The model under review builds one solid part; all positions refer to its coordinate system, in mm. Face numbers are marked on the shaded views. A direction names the side the tool comes from. Coordinates: 2 decimals unless noted, no trailing zeros. Order: outer loops, then holes, each group sorted by start corner. A loop starts at its lowest first (then second) coordinate and runs counter-clockwise, first axis right, second up. Notation, with made-up numbers: M -19.75,40.5 L 15.25,40.5 A31 cw 15.25,65.5 Z; hole C 47.25,45.5 d7. An arc over 180 degrees is marked long. One line per item, written item: value.
```python
from build123d import *

# Parameters (mm, degrees)
SKETCH_1_R          = 1.5
EXTRUDE_1_DEPTH     = 6
SKETCH_2_R          = 3.5
EXTRUDE_2_DEPTH     = 1.8
CUT_EXTRUDE_1_DEPTH = 1
FILLET_1_R          = 1


with BuildPart() as part:
    # 草图1 → 凸台-拉伸1 (new body)
    with BuildSketch(Plane(origin=(0, 0, 0), x_dir=(1, 0, 0), z_dir=(0, 1, 0))):
        with Locations(Location((0, 0, 0), (0, 0, 270))):
            Circle(SKETCH_1_R)
    extrude(amount=EXTRUDE_1_DEPTH)

    # 草图2 → 凸台-拉伸2 (add)
    with BuildSketch(Plane.XZ):
        with Locations(Location((0, 0, 0), (0, 0, 270))):
            Circle(SKETCH_2_R)
    extrude(amount=EXTRUDE_2_DEPTH)

    # 草图3 → 切除-拉伸1 (cut)
    with BuildSketch(Plane.XZ.offset(1.8)):
        Polygon((1, 0.577350269), (0, 1.154700538), (-1, 0.577350269), (-1, -0.577350269), (0, -1.154700538), (1, -0.577350269), align=None)
    extrude(amount=-CUT_EXTRUDE_1_DEPTH, mode=Mode.SUBTRACT)

    # 圆角1
    fillet_1_edges = [part.edges().sort_by_distance(p)[0] for p in [
        (0, -1.8, 3.5),
    ]]
    fillet(fillet_1_edges, radius=FILLET_1_R)


solid = part.part
```
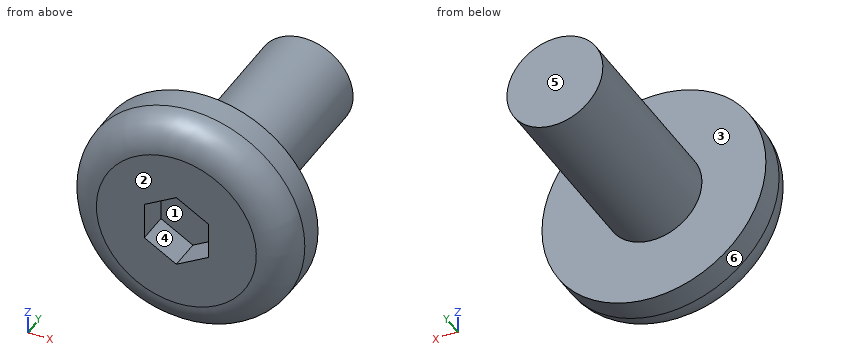
(1) Mouldability with a two-part tool opening along X and no side actions: class the marked faces 4, 5 and 6 as +X half, -X half, draft (parallel to the pull), parting line (faces both ways), or undercut.
Geometry results:
face 4: undercut
face 5: draft
face 6: parting line
(2) For L1, parallel to X at y = 3.5, z = 0; L2, parallel to Y at x = -2.25, z = 1.25; L3, parallel to Z at x = -0.25, y = 0.75, list the stretches that pass through material, from the lowest coordinate up.
Geometry results:
L1: x = -1.5 to 1.5
L2: y = -1.8 to 0
L3: z = -1.48 to 1.48
(3) We need section B-B, the plane y = 4.25. State the section outline as (x, z) points.
Geometry results:
outline: C 0,0 d3
(4) Tool access review of the marked faces 1, 2 and 3: name each direction out of +Z, -Z, +X, -X, +Y, -Y from which nothing blocks a thin tool from reaching the whole face with its end or side.
Geometry results:
face 1: -Y
face 2: +Z, -Z, +X, -X, -Y
face 3: +Y
(5) Insertion check: pin 1 Ø0.6 at (x, z) = (0, 0) entering from -Y. The pin has a flat end and moves straight along its axis. Give the tip position at first contact, or say it passes through.
Geometry results:
pin 1: stops at y = -0.8
(6) We need section A-A, the plane z = 0. State the section outline as (x, y) points, plus the area to 3 significant figures.
Geometry results:
outline: M -3.5,-0.8 A1 ccw -2.5,-1.8 L -1,-1.8 L -1,-0.8 L 1,-0.8 L 1,-1.8 L 2.5,-1.8 A1 ccw 3.5,-0.8 L 3.5,0 L 1.5,0 L 1.5,6 L -1.5,6 L -1.5,0 L -3.5,0 Z
area: 28.2 mm2
